Design review of the part built by this model. Coordinates are the model's own, in mm. Face numbers are marked on the shaded views. A direction names the side the tool comes from. Coordinates: 2 decimals unless noted, no trailing zeros. Write each loop counter-clockwise with the first axis right and the second up, starting at its lowest first coordinate (ties: lowest second). Pieces come first, ordered by that corner, then holes. Notation, with made-up numbers: (-29, 84.25) -> (-16, 84.25) arc R18 ccw to (-16, 113.25) -> close; hole circle Ø8 at (62.5, -33). An arc over 180 degrees is marked (long way). Answer in a Markdown table with one row per item. Add a question column.
Item 1: Take a section at C-C, the plane z = 1.75. Write out the cut boundary in (x, y), and give its area (3 significant figures).
Item 2: To check wall thickness, follow line 1 (Y direction, x = 0, z = 0.1); line 2 (Y direction, x = 0, z = -2.1); line 3 (Z direction, x = 3.5, y = 10.5). State the ranges of each line that lie inside material, in increasing order.
Item 3: Take a section at D-D, the plane x = -4.5. Write out the cut boundary in (y, z), and give its area (3 significant figures).
Item 4: Take a section at A-A, the plane x = 0. Write out the cut boundary in (y, z).
Item 5: Draft analysis for pull direction X (two halves, no side actions). For the marked faces 4, 5 and 6, state which applies: released by +X, released by -X, zero draft, split by the parting line, or undercut.
Item 6: For the marked faces 1, 2 and 3, list the 3-axis set-ups (+Z, -Z, +X, -X, +Y, -Y) from which the entire face can be reached by the end or side of a thin tool; tool diameter is ignored.
Item 7: Clearance check with flat-ended pins moving along their axes: P1, Ø3, axis at x = 7.5, y = 10, coming from the +Z side; P2, Ø6, axis at x = -8.5, z = 4, coming from the +Y side; P3, Ø2, axis at y = -0.5, z = 1, coming from the +X side; P4, Ø6, axis at x = 6.5, y = -7, coming from the -Z side. State where each tip first meets the part, or that it passes through.
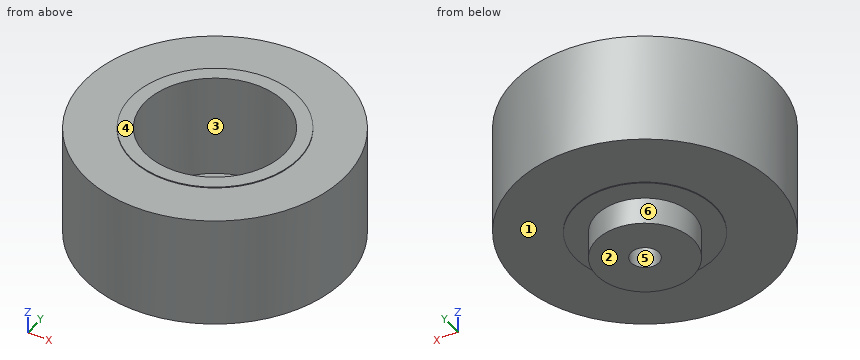
from build123d import *

# Parameters (mm, degrees)
CROQUIS1_R                   = 9
CROQUIS1_R_2                 = 7.5
SALIENTE_EXTRUIR1_DEPTH      = 12
SALIENTE_EXTRUIR2_DEPTH      = 1
SALIENTE_EXTRUIR2_DEPTH_BACK = 0.1
CROQUIS2_R                   = 7.5
CROQUIS3_R                   = 5.2
CROQUIS3_R_2                 = 1.5
SALIENTE_EXTRUIR4_DEPTH      = 3
CROQUIS4_R                   = 14
CROQUIS4_R_2                 = 9
SALIENTE_EXTRUIR5_DEPTH      = 11.9
CORTAR_EXTRUIR1_START        = -15
CROQUIS6_R                   = 1.5
CORTAR_EXTRUIR1_DEPTH        = 15


with BuildPart() as part:
    # Croquis1 → Saliente-Extruir1 (new body)
    with BuildSketch(Plane.XY):
        Circle(CROQUIS1_R)
        Circle(CROQUIS1_R_2, mode=Mode.SUBTRACT)
    extrude(amount=SALIENTE_EXTRUIR1_DEPTH)

    # Croquis2 → Saliente-Extruir2 (add, two sides: drawn at the far end of the back side and taken through both)
    with BuildSketch(Plane.XY.offset(-SALIENTE_EXTRUIR2_DEPTH_BACK)):
        Circle(CROQUIS2_R)
    extrude(amount=SALIENTE_EXTRUIR2_DEPTH + SALIENTE_EXTRUIR2_DEPTH_BACK)

    # Croquis3 → Saliente-Extruir4 (add)
    with BuildSketch(Plane.XY):
        Circle(CROQUIS3_R)
        Circle(CROQUIS3_R_2, mode=Mode.SUBTRACT)
    extrude(amount=-SALIENTE_EXTRUIR4_DEPTH)

    # Croquis4 → Saliente-Extruir5 (add)
    with BuildSketch(Plane(origin=(0, 0, 0), x_dir=(-1, 0, 0), z_dir=(0, 0, -1))):
        Circle(CROQUIS4_R)
        Circle(CROQUIS4_R_2, mode=Mode.SUBTRACT)
    extrude(amount=-SALIENTE_EXTRUIR5_DEPTH)

    # Croquis6 → Cortar-Extruir1 (cut)
    with BuildSketch(Plane(origin=(0, 0, -3), x_dir=(-1, 0, 0), z_dir=(0, 0, -1)).offset(CORTAR_EXTRUIR1_START)):
        with Locations(Location((0, 0, 0), (0, 0, 180))):
            Circle(CROQUIS6_R)
    extrude(amount=CORTAR_EXTRUIR1_DEPTH, mode=Mode.SUBTRACT)


solid = part.part
Answers:
| question | item | result |
|---|---|---|
| 1 | outline | circle Ø28 at (0, 0); hole circle Ø15 at (0, 0) |
| 1 | area | 439 mm^2 |
| 2 | line 1 | y = -14 to -1.5, 1.5 to 14 |
| 2 | line 2 | y = -5.2 to -1.5, 1.5 to 5.2 |
| 2 | line 3 | z = 0 to 11.9 |
| 3 | outline | (-13.26, 0) -> (-6, 0) -> (-6, -0.1) -> (-2.61, -0.1) -> (-2.61, -3) -> (2.61, -3) -> (2.61, -0.1) -> (6, -0.1) -> (6, 0) -> (13.26, 0) -> (13.26, 11.9) -> (7.79, 11.9) -> (7.79, 12) -> (6, 12) -> (6, 1) -> (-6, 1) -> (-6, 12) -> (-7.79, 12) -> (-7.79, 11.9) -> (-13.26, 11.9) -> close |
| 3 | area | 201 mm^2 |
| 4 | outline | (-14, 0) -> (-7.5, 0) -> (-7.5, -0.1) -> (-5.2, -0.1) -> (-5.2, -3) -> (-1.5, -3) -> (-1.5, 1) -> (-7.5, 1) -> (-7.5, 12) -> (-9, 12) -> (-9, 11.9) -> (-14, 11.9) -> close; (1.5, -3) -> (5.2, -3) -> (5.2, -0.1) -> (7.5, -0.1) -> (7.5, 0) -> (14, 0) -> (14, 11.9) -> (9, 11.9) -> (9, 12) -> (7.5, 12) -> (7.5, 1) -> (1.5, 1) -> close |
| 5 | face 4 | zero draft |
| 5 | face 5 | undercut |
| 5 | face 6 | split by the parting line |
| 6 | face 1 | -Z |
| 6 | face 2 | -Z, +X, -X, +Y, -Y |
| 6 | face 3 | +Z |
| 7 | P1 | stops at z = 11.9 |
| 7 | P2 | stops at y = 12.87 |
| 7 | P3 | stops at x = 14 |
| 7 | P4 | stops at z = -0.1 |
